For this review, take the finished solid that the model builds, in its own axes (mm). Round coordinates to 2 decimals unless told otherwise and drop trailing zeros. Order: outer loops, then holes, each group sorted by start corner. A loop starts at its lowest first (then second) coordinate and runs counter-clockwise, first axis right, second up. Notation, with made-up numbers: M 28,-3.75 L 78,-3.75 A27 ccw 78,12.25 Z; hole C 21.25,46.25 d6. An arc over 180 degrees is marked long. Use a Markdown table: item, result.
from build123d import *

# Parameters (mm, degrees)
SKETCH1_W                = 117
SKETCH1_H                = 8
BOSS_EXTRUDE1_DEPTH      = 3.8
SKETCH2_R                = 1.75
CUT_EXTRUDE4_DEPTH       = 59.759594961
FILLET1_R                = 4
FILLET2_R                = 1.5
BOSS_EXTRUDE2_DEPTH      = 2
BOSS_EXTRUDE2_DEPTH_BACK = 5.8
SKETCH3_W                = 55
SKETCH3_H                = 2
FILLET3_R                = 2
FILLET4_R                = 2
FILLET5_R                = 1


with BuildPart() as part:
    # Sketch1 → Boss-Extrude1 (new body)
    with BuildSketch(Plane(origin=(0, 0, 0), x_dir=(1, 0, 0), z_dir=(0, 1, 0))):
        Rectangle(SKETCH1_W, SKETCH1_H)
    extrude(amount=BOSS_EXTRUDE1_DEPTH)

    # Sketch2 → Cut-Extrude4 (cut, through all)
    with BuildSketch(Plane(origin=(0, 3.8, 0), x_dir=(1, 0, 0), z_dir=(0, 1, 0))):
        with Locations(Location((-54.75, 0, 0), (0, 0, 270))):
            Circle(SKETCH2_R)
        with Locations(Location((54.75, 0, 0), (0, 0, 270))):
            Circle(SKETCH2_R)
    extrude(amount=-CUT_EXTRUDE4_DEPTH, mode=Mode.SUBTRACT)

    # Fillet1
    fillet1_edges = [part.edges().sort_by_distance(p)[0] for p in [
        (58.5, 1.9, -4),
        (58.5, 1.9, 4),
        (-58.5, 1.9, 4),
        (-58.5, 1.9, -4),
    ]]
    fillet(fillet1_edges, radius=FILLET1_R - 0.0001)  # a hair under: the kernel refuses the full size

    # Fillet2
    fillet2_edges = [part.edges().sort_by_distance(p)[0] for p in [
        (0, 0, -4),
        (0, 3.8, -4),
        (0, 0, 4),
        (-57.328456414, 0, -2.828456414),
        (-57.328456414, 0, 2.828456414),
        (57.328456414, 0, 2.828456414),
        (57.328456414, 0, -2.828456414),
        (0, 3.8, 4),
        (-57.328456414, 3.8, -2.828456414),
        (-57.328456414, 3.8, 2.828456414),
        (57.328456414, 3.8, 2.828456414),
        (57.328456414, 3.8, -2.828456414),
    ]]
    fillet(fillet2_edges, radius=FILLET2_R)

    # Sketch3 → Boss-Extrude2 (add, two sides: drawn at the far end of the back side and taken through both)
    with BuildSketch(Plane(origin=(0, 3.8, 0), x_dir=(1, 0, 0), z_dir=(0, 1, 0)).offset(-BOSS_EXTRUDE2_DEPTH_BACK)):
        Rectangle(SKETCH3_W, SKETCH3_H)
    extrude(amount=BOSS_EXTRUDE2_DEPTH + BOSS_EXTRUDE2_DEPTH_BACK)

    # Fillet3
    fillet3_edges = [part.edges().sort_by_distance(p)[0] for p in [
        (-27.5, 0, 0),
        (27.5, 0, 0),
        (-27.5, 3.8, 0),
        (27.5, 3.8, 0),
    ]]
    fillet(fillet3_edges, radius=FILLET3_R - 0.0001)  # a hair under: the kernel refuses the full size

    # Fillet4
    fillet4_edges = [part.edges().sort_by_distance(p)[0] for p in [
        (27.5, -2, 0),
        (-27.5, -2, 0),
        (27.5, 5.8, 0),
        (-27.5, 5.8, 0),
    ]]
    fillet(fillet4_edges, radius=FILLET4_R)

    # Fillet5
    fillet5_edges = [part.edges().sort_by_distance(p)[0] for p in [
        (0, 3.8, -1),
        (0, 3.8, 1),
        (0, 0, 1),
        (0, 0, -1),
    ]]
    fillet(fillet5_edges, radius=FILLET5_R - 0.0001)  # a hair under: the kernel refuses the full size


solid = part.part
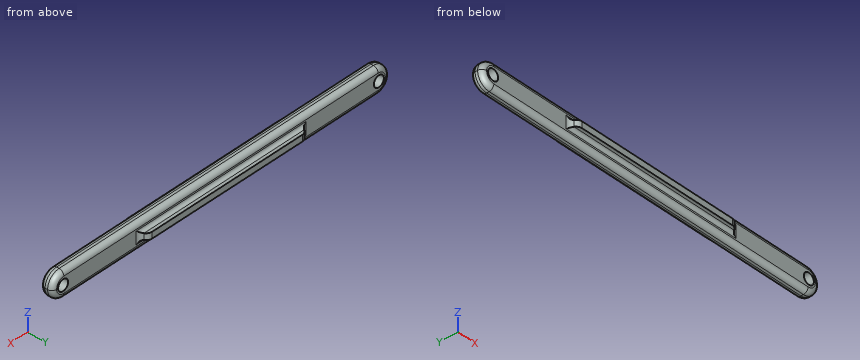
Q1. Add section A-A (x = -3.5). Write out the cut boundary in (y, z), then the cut area to 3 significant figures.
Determined:
| item | result |
|---|---|
| outline | M -2,-1 L -1,-1 A1 cw 0,-2 L 0,-2.5 A1.5 ccw 1.5,-4 L 2.3,-4 A1.5 ccw 3.8,-2.5 L 3.8,-2 A1 cw 4.8,-1 L 5.8,-1 L 5.8,1 L 4.8,1 A1 cw 3.8,2 L 3.8,2.5 A1.5 ccw 2.3,4 L 1.5,4 A1.5 ccw 0,2.5 L 0,2 A1 cw -1,1 L -2,1 Z |
| area | 37.3 mm^2 |
Q2. Clearance check with flat-ended pins moving along their axes: pin 1 (1.1 mm diameter, centred on x = 7.5, y = -1.5, fed in from -Z); pin 2 (1.5 mm diameter, centred on x = -26.5, y = 0, fed in from +Z); pin 3 (4.5 mm diameter, centred on x = -54.75, z = 0, fed in from +Y); pin 4 (3 mm diameter, centred on x = 54.75, z = 0, fed in from +Y). State where each tip first meets the part, or that it passes through.
Determined:
| item | result |
|---|---|
| pin 1 | stops at z = -1 |
| pin 2 | stops at z = 3.8 |
| pin 3 | stops at y = 3.8 |
| pin 4 | passes through |
Q3. Wall thickness on line 1 along X through (y, z) = (3, 0.25); line 2 along X through (y, z) = (1.1, 0); line 3 along Y through (x, z) = (48, 2): over which ranges is each line inside the solid? List them lowest first. Write a range as [from, to].
Determined:
| item | result |
|---|---|
| line 1 | x = [-58.32, -56.48], [-53.02, 53.02], [56.48, 58.32] |
| line 2 | x = [-58.45, -56.5], [-53, 53], [56.5, 58.45] |
| line 3 | y = [0, 3.8] |
Q4. Add section B-B (x = 41.5). Write out the cut boundary in (y, z).
Determined:
| item | result |
|---|---|
| outline | M 0,-2.5 A1.5 ccw 1.5,-4 L 2.3,-4 A1.5 ccw 3.8,-2.5 L 3.8,2.5 A1.5 ccw 2.3,4 L 1.5,4 A1.5 ccw 0,2.5 Z |
